Build history of the part. All positions in model axes, mm. A direction names the side the tool comes from. Round coordinates to 2 decimals unless told otherwise and drop trailing zeros. Loops run counter-clockwise (first coordinate to the right, second up) from the corner with the lowest first, then second, coordinate; pieces in that order, holes last. Notation, with made-up numbers: M -39.75,-37 L -4.75,-37 A27 cw -4.75,-9 Z; hole C -32.75,46 d5. An arc over 180 degrees is marked long. One line per item, written item: value.
```python
from build123d import *

# Parameters (mm, degrees)
CROQUIS1_W              = 8
CROQUIS1_H              = 8
EXTRUIR1_DEPTH          = 40
CORTAR_EXTRUIR3_DEPTH   = 8
CROQUIS5_R              = 4
SALIENTE_EXTRUIR1_DEPTH = 44.25


with BuildPart() as part:
    # Croquis1 → Extruir1 (new body)
    with BuildSketch(Plane.XY):
        Rectangle(CROQUIS1_W, CROQUIS1_H)
    extrude(amount=EXTRUIR1_DEPTH)

    # Croquis4 → Cortar-Extruir3 (cut)
    with BuildSketch(Plane(origin=(4, 0, 0), x_dir=(0, 0, -1), z_dir=(1, 0, 0))):
        Polygon((-36.96, -4), (-36.6612042, -2.884878893), (-36.21598653, -2.884878893), (-35.91719073, -4), align=None)
        Polygon((-39, -4), (-38.7012042, -2.884878893), (-38.25598653, -2.884878893), (-37.95719073, -4), align=None)
        Polygon((-34.92, -4), (-34.6212042, -2.884878893), (-34.17598653, -2.884878893), (-33.87719073, -4), align=None)
        Polygon((-32.88, -4), (-32.5812042, -2.884878893), (-32.13598653, -2.884878893), (-31.83719073, -4), align=None)
        Polygon((-30.84, -4), (-30.5412042, -2.884878893), (-30.09598653, -2.884878893), (-29.79719073, -4), align=None)
        Polygon((-28.8, -4), (-28.5012042, -2.884878893), (-28.05598653, -2.884878893), (-27.75719073, -4), align=None)
        Polygon((-26.76, -4), (-26.4612042, -2.884878893), (-26.01598653, -2.884878893), (-25.71719073, -4), align=None)
        Polygon((-24.72, -4), (-24.4212042, -2.884878893), (-23.97598653, -2.884878893), (-23.67719073, -4), align=None)
        Polygon((-22.68, -4), (-22.3812042, -2.884878893), (-21.93598653, -2.884878893), (-21.63719073, -4), align=None)
        Polygon((-20.64, -4), (-20.3412042, -2.884878893), (-19.89598653, -2.884878893), (-19.59719073, -4), align=None)
        Polygon((-18.6, -4), (-18.3012042, -2.884878893), (-17.85598653, -2.884878893), (-17.55719073, -4), align=None)
        Polygon((-16.56, -4), (-16.2612042, -2.884878893), (-15.81598653, -2.884878893), (-15.51719073, -4), align=None)
        Polygon((-14.52, -4), (-14.2212042, -2.884878893), (-13.77598653, -2.884878893), (-13.47719073, -4), align=None)
        Polygon((-12.48, -4), (-12.1812042, -2.884878893), (-11.73598653, -2.884878893), (-11.43719073, -4), align=None)
        Polygon((-10.44, -4), (-10.1412042, -2.884878893), (-9.69598653, -2.884878893), (-9.39719073, -4), align=None)
        Polygon((-8.4, -4), (-8.1012042, -2.884878893), (-7.65598653, -2.884878893), (-7.35719073, -4), align=None)
        Polygon((-6.36, -4), (-6.0612042, -2.884878893), (-5.61598653, -2.884878893), (-5.31719073, -4), align=None)
        Polygon((-4.32, -4), (-4.0212042, -2.884878893), (-3.57598653, -2.884878893), (-3.27719073, -4), align=None)
        Polygon((-2.28, -4), (-1.9812042, -2.884878893), (-1.53598653, -2.884878893), (-1.23719073, -4), align=None)
    extrude(amount=-CORTAR_EXTRUIR3_DEPTH, mode=Mode.SUBTRACT)

    # Croquis5 → Saliente-Extruir1 (add)
    with BuildSketch(Plane.XY.offset(40)):
        Circle(CROQUIS5_R)
    extrude(amount=SALIENTE_EXTRUIR1_DEPTH)


solid = part.part
```
Item 1: Slice it at B-B, the plane z = 56.5. Give the cut face in (x, y).
Check values:
outline: C 0,0 d8
Item 2: Drop flat-ended pins along their axis: P1, Ø2, axis at x = 1, y = -1, coming from the -Z side; P2, Ø2, axis at x = 2, z = 60, coming from the -Y side. Give the stop position or say it passes through.
Check values:
P1: stops at z = 0
P2: stops at y = -3.87
Item 3: Which spindle directions (+Z, -Z, +X, -X, +Y, -Y) get a long thin tool onto all of the face, cutting with end or side? Do faces 1 (the face through (-0.867, -3.905, 61.815)), 2 (the face through (3, 3, 40)), 3 (the face through (3, -3, 40)). Say none if no direction does.
Check values:
face 1: +Z
face 2: +Z, +X, +Y
face 3: +Z, +X, -Y
Item 4: Slice it at A-A, the plane y = 1. Give the cut face in (x, z).
Check values:
outline: M -4,0 L 4,0 L 4,40 L 3.87,40 L 3.87,84.25 L -3.87,84.25 L -3.87,40 L -4,40 Z
Item 5: Wall check: line 1 along Y through (x, z) = (-0.25, 79); line 2 along Z through (x, y) = (-2.75, 3.5); line 3 along Y through (x, z) = (-0.75, 58.5). Give the ranges that are in metal, low to high.
Check values:
line 1: y = -3.99 to 3.99
line 2: z = 0 to 40
line 3: y = -3.93 to 3.93
